from build123d import *

# Parameters (mm, degrees)
SKETCH1_W                   = 90
SKETCH1_H                   = 290
BASE_FLANGE1_DEPTH          = 3
SM_EDGE_FLANGE_1_DEPTH      = 290
SM_EDGE_FLANGE_1_BEND_DEPTH = 290
INDENT1_START               = 23
INDENT1_DEPTH               = 104
INDENT1_START_2             = 26.270388893
INDENT1_2_DEPTH             = 97.459222009
INDENT1_3_DEPTH             = 0.729611107
INDENT1_START_3             = 123
INDENT1_4_DEPTH             = 0.729610902
INDENT1_START_4             = 119.9999999
INDENT1_5_DEPTH             = 6.0000001
INDENT1_START_5             = 24
INDENT1_6_DEPTH             = 6
INDENT1_START_6             = -290
INDENT1_7_DEPTH             = 6.65
INDENT2_START               = 23
INDENT2_DEPTH               = 104
INDENT2_START_2             = -11.0000001
INDENT2_2_DEPTH             = 11.0000001
INDENT2_START_3             = 24
INDENT2_3_DEPTH             = 102
CUT_EXTRUDE1_DEPTH          = 317.754179273
CUT_EXTRUDE1_DEPTH_BACK     = 317.754179273
SKETCH15_R                  = 4.2
CUT_EXTRUDE2_DEPTH          = 317.754179273
CUT_EXTRUDE2_DEPTH_BACK     = 317.754179273


with BuildPart() as part:
    # Base-Flange1: sheet metal written as solids
    # Sketch1 → Base-Flange1 (new body)
    with BuildSketch(Plane(origin=(0, 207.95, 0), x_dir=(1, 0, 0), z_dir=(0, 1, 0))):
        with Locations((75, 145)):
            Rectangle(SKETCH1_W, SKETCH1_H)
    extrude(amount=-BASE_FLANGE1_DEPTH)

    # 邊線-凸緣1: sheet metal written as solids
    # 邊線-凸緣1 section (on a plane across the edge) → 邊線-凸緣1 (add)
    with BuildSketch(Plane(origin=(27, 204.95, 0), x_dir=(1, 0, 0), z_dir=(0, 0, -1))):
        with BuildLine():
            Line((-3, 3), (-3, 15.9))
            Line((-3, 15.9), (0, 15.9))
            Line((0, 15.9), (0, 3))
            ThreePointArc((0, 3), (0.878679656, 0.878679656), (3, 0))
            Line((3, 0), (3, -3))
            ThreePointArc((3, -3), (-1.242640687, -1.242640687), (-3, 3))
        make_face()
    extrude(amount=SM_EDGE_FLANGE_1_DEPTH)

    # 邊線-凸緣1 section 2 (on a plane across the edge) → 邊線-凸緣1 bend (add)
    with BuildSketch(Plane(origin=(123, 204.95, -290), x_dir=(-1, 0, 0), z_dir=(0, 0, 1))):
        with BuildLine():
            Line((-3, 3), (-3, 15.9))
            Line((-3, 15.9), (0, 15.9))
            Line((0, 15.9), (0, 3))
            ThreePointArc((0, 3), (0.878679656, 0.878679656), (3, 0))
            Line((3, 0), (3, -3))
            ThreePointArc((3, -3), (-1.242640687, -1.242640687), (-3, 3))
        make_face()
    extrude(amount=SM_EDGE_FLANGE_1_BEND_DEPTH)

    # Indent1: read off the stored shape, not the designer's step
    # Indent1 outline → Indent1 (cut)
    with BuildSketch(Plane.YZ.offset(INDENT1_START)):
        with BuildLine():
            Line((192.05, -290), (207.95, -290))
            ThreePointArc((207.95, -290), (200, -282.05), (192.05, -290))
        make_face()
    extrude(amount=INDENT1_DEPTH, mode=Mode.SUBTRACT)

    # Indent2: read off the stored shape, not the designer's step
    # Indent2 outline → Indent2 (cut)
    with BuildSketch(Plane.YZ.offset(INDENT2_START)):
        with BuildLine():
            ThreePointArc((189.05, -6.433311744), (197.7062633, -12.491147744), (207.950014124, -9.903902031))
            Line((207.950014124, -9.903902031), (209, -9.061062257))
            Line((209, -9.061062257), (209, 1))
            Line((209, 1), (188, 1))
            Line((188, 1), (188, 0))
            Line((188, 0), (188, -4.64612958))
            Line((188, -4.64612958), (189.05, -6.433311744))
        make_face()
    extrude(amount=INDENT2_DEPTH, mode=Mode.SUBTRACT)

    # Sketch15 → Cut-Extrude1 (cut, two sides: drawn at the far end of the back side and taken through both)
    with BuildSketch(Plane(origin=(0, 207.95, 0), x_dir=(1, 0, 0), z_dir=(0, 1, 0)).offset(-CUT_EXTRUDE1_DEPTH_BACK)):
        with Locations((41.5, 270.8)):
            Circle(SKETCH15_R)
        with Locations((108.5, 270.8)):
            Circle(SKETCH15_R)
        with Locations((41.5, 250.8)):
            Circle(SKETCH15_R)
        with Locations((108.5, 250.8)):
            Circle(SKETCH15_R)
        with Locations((41.5, 230.8)):
            Circle(SKETCH15_R)
        with Locations((108.5, 230.8)):
            Circle(SKETCH15_R)
        with Locations((41.5, 210.8)):
            Circle(SKETCH15_R)
        with Locations((108.5, 210.8)):
            Circle(SKETCH15_R)
        with Locations((41.5, 190.8)):
            Circle(SKETCH15_R)
        with Locations((108.5, 190.8)):
            Circle(SKETCH15_R)
        with Locations((41.5, 170.8)):
            Circle(SKETCH15_R)
        with Locations((108.5, 170.8)):
            Circle(SKETCH15_R)
        with Locations((41.5, 150.8)):
            Circle(SKETCH15_R)
        with Locations((108.5, 150.8)):
            Circle(SKETCH15_R)
        with Locations((41.5, 130.8)):
            Circle(SKETCH15_R)
        with Locations((108.5, 130.8)):
            Circle(SKETCH15_R)
        with Locations((41.5, 110.8)):
            Circle(SKETCH15_R)
        with Locations((108.5, 110.8)):
            Circle(SKETCH15_R)
        with Locations((41.5, 90.8)):
            Circle(SKETCH15_R)
        with Locations((108.5, 90.8)):
            Circle(SKETCH15_R)
        with Locations((41.5, 70.8)):
            Circle(SKETCH15_R)
        with Locations((108.5, 70.8)):
            Circle(SKETCH15_R)
    extrude(amount=CUT_EXTRUDE1_DEPTH + CUT_EXTRUDE1_DEPTH_BACK, mode=Mode.SUBTRACT)

    # Sketch16 → Cut-Extrude2 (cut, two sides: drawn at the far end of the back side and taken through both)
    with BuildSketch(Plane(origin=(0, 207.95, 0), x_dir=(1, 0, 0), z_dir=(0, 1, 0)).offset(-CUT_EXTRUDE2_DEPTH_BACK)):
        with BuildLine():
            Line((55, 54.903913368), (55, 124.903913368))
            ThreePointArc((55, 124.903913368), (75, 144.903913368), (95, 124.903913368))
            Line((95, 124.903913368), (95, 54.903913368))
            ThreePointArc((95, 54.903913368), (75, 34.903913368), (55, 54.903913368))
        make_face()
    extrude(amount=CUT_EXTRUDE2_DEPTH + CUT_EXTRUDE2_DEPTH_BACK, mode=Mode.SUBTRACT)


with BuildPart() as body_2:
    # Indent1 2 outline → Indent1 2 (new body)
    with BuildSketch(Plane.YZ.offset(INDENT1_START_2)):
        with BuildLine():
            Line((204.95, -285.559279338), (204.95, -290))
            Line((204.95, -290), (206.65, -290))
            ThreePointArc((206.65, -290), (206.210475022, -287.622501314), (204.95, -285.559279338))
        make_face()
    extrude(amount=INDENT1_2_DEPTH)

    # Indent1 3 outline → Indent1 3 (add)
    with BuildSketch(Plane.YZ.offset(INDENT1_START_2)):
        with BuildLine():
            Line((193.35, -290), (204.95, -290))
            Line((204.95, -290), (204.95, -285.559279338))
            ThreePointArc((204.95, -285.559279338), (197.622501314, -283.789524978), (193.35, -290))
        make_face()
    extrude(amount=INDENT1_3_DEPTH)

    # Indent1 4 outline → Indent1 4 (add)
    with BuildSketch(Plane.YZ.offset(INDENT1_START_3)):
        with BuildLine():
            Line((193.35, -290), (204.95, -290))
            Line((204.95, -290), (204.95, -285.559279338))
            ThreePointArc((204.95, -285.559279338), (197.622501314, -283.789524978), (193.35, -290))
        make_face()
    extrude(amount=INDENT1_4_DEPTH)

    # Indent1 5 outline → Indent1 5 (add)
    with BuildSketch(Plane.YZ.offset(INDENT1_START_4)):
        with BuildLine():
            Line((193.35, -290), (206.65, -290))
            ThreePointArc((206.65, -290), (200, -283.35), (193.35, -290))
        make_face()
    extrude(amount=INDENT1_5_DEPTH)

    # Indent1 6 outline → Indent1 6 (add)
    with BuildSketch(Plane.YZ.offset(INDENT1_START_5)):
        with BuildLine():
            Line((193.35, -290), (206.65, -290))
            ThreePointArc((206.65, -290), (200, -283.35), (193.35, -290))
        make_face()
    extrude(amount=INDENT1_6_DEPTH)

    # Indent1 7 outline → Indent1 7 (cut)
    with BuildSketch(Plane.XY.offset(INDENT1_START_6)):
        with BuildLine():
            Line((123, 192), (123, 201.95))
            ThreePointArc((123, 201.95), (122.121320344, 204.071320344), (120, 204.95))
            Line((120, 204.95), (119.9999999, 192))
            Line((119.9999999, 192), (123, 192))
        make_face()
        with BuildLine():
            Line((27, 192), (30, 192))
            Line((30, 192), (30, 204.95))
            ThreePointArc((30, 204.95), (27.878679656, 204.071320344), (27, 201.95))
            Line((27, 201.95), (27, 192))
        make_face()
        with BuildLine():
            ThreePointArc((123.729603466, 206.650006169), (125.402666971, 204.559825589), (126, 201.95))
            Line((126, 201.95), (126, 208))
            Line((126, 208), (122.028355761, 208))
            Line((122.028355761, 208), (123.729603466, 206.650006169))
        make_face()
        with BuildLine():
            Line((24, 208), (24, 201.95))
            ThreePointArc((24, 201.95), (24.597331636, 204.559822705), (26.270391517, 206.650002187))
            Line((26.270391517, 206.650002187), (27.971640511, 208))
            Line((27.971640511, 208), (24, 208))
        make_face()
    extrude(amount=INDENT1_7_DEPTH, mode=Mode.SUBTRACT)


with BuildPart() as body_3:
    # Indent2 2 outline → Indent2 2 (new body)
    with BuildSketch(Plane.XY.offset(INDENT2_START_2)):
        with BuildLine():
            Line((24, 201.95), (24, 189.05))
            Line((24, 189.05), (27, 189.05))
            Line((27, 189.05), (27, 201.95))
            ThreePointArc((27, 201.95), (27.878679656, 204.071320344), (30, 204.95))
            Line((30, 204.95), (120, 204.95))
            ThreePointArc((120, 204.95), (122.121320344, 204.071320344), (123, 201.95))
            Line((123, 201.95), (123, 189.05))
            Line((123, 189.05), (126, 189.05))
            Line((126, 189.05), (126, 201.95))
            ThreePointArc((126, 201.95), (124.242640687, 206.192640687), (120, 207.95))
            Line((120, 207.95), (30, 207.95))
            ThreePointArc((30, 207.95), (25.757359313, 206.192640687), (24, 201.95))
        make_face()
    extrude(amount=INDENT2_2_DEPTH)

    # Indent2 3 outline → Indent2 3 (cut)
    with BuildSketch(Plane.YZ.offset(INDENT2_START_3)):
        with BuildLine():
            Line((207.95, -11.0000001), (207.950016725, -7.602449216))
            ThreePointArc((207.950016725, -7.602449216), (204.322791843, -10.115012145), (200.000000001, -11))
            Line((200.000000001, -11), (207.95, -11.0000001))
        make_face()
        with BuildLine():
            Line((189.05, -11.0000001), (200.000000001, -11))
            ThreePointArc((200.000000001, -11), (192.601479194, -8.140140655), (189.05, -1.047616342))
            Line((189.05, -1.047616342), (189.05, -11.0000001))
        make_face()
    extrude(amount=INDENT2_3_DEPTH, mode=Mode.SUBTRACT)


solid = part.part
Here's how the part is built. I have some questions about the finished solid (model axes, mm). A direction names the side the tool comes from. Coordinates: 2 decimals unless noted, no trailing zeros. Write each loop counter-clockwise with the first axis right and the second up, starting at its lowest first coordinate (ties: lowest second). Pieces come first, ordered by that corner, then holes.
1) I'm going to push flat-ended pins straight in: pin 1 (11 mm diameter, centred on x = 41.5, z = -150.8, fed in from +Y); pin 2 (0.9 mm diameter, centred on y = 206.5, z = -82, fed in from +X); pin 3 (1 mm diameter, centred on x = 76.5, z = -243, fed in from -Y); pin 4 (1.5 mm diameter, centred on y = 207, z = -105, fed in from -X). Where does each tip first touch, or does it pass through?
Filled in:
pin 1: stops at y = 207.95
pin 2: stops at x = 124.38
pin 3: stops at y = 204.95
pin 4: stops at x = 25.82
2) If we section it at D-D (x = 67): List the corners of the cut face in (y, z) for me, plus the area to 3 significant figures.
Filled in:
outline: (204.95, -283.78) arc R7.95 cw to (207.95, -290) - (207.95, -143.23) - (204.95, -143.23) - close; (204.95, -36.57) - (207.95, -36.57) - (207.95, -9.9) arc R12.7 cw to (204.95, -11.7) - close
area: 504 mm2
3) If we section it at B-B (y = 196): List the corners of the cut face in (x, z) for me, plus the area to 3 significant figures.
Filled in:
outline: (24, -283.13) - (27, -283.13) - (27, -12.05) - (24, -12.05) - close; (123, -283.13) - (126, -283.13) - (126, -12.05) - (123, -12.05) - close
area: 1,630 mm2
4) If we section it at C-C (z = -44.5): List the corners of the cut face in (x, y) for me.
Filled in:
outline: (24, 189.05) - (27, 189.05) - (27, 201.95) arc R3 cw to (30, 204.95) - (57.92, 204.95) - (57.92, 207.95) - (30, 207.95) arc R6 ccw to (24, 201.95) - close; (92.08, 204.95) - (120, 204.95) arc R3 cw to (123, 201.95) - (123, 189.05) - (126, 189.05) - (126, 201.95) arc R6 ccw to (120, 207.95) - (92.08, 207.95) - close
5) If we section it at A-A (z = -170.8): List the corners of the cut face in (x, y) for me, plus the area to 3 significant figures.
Filled in:
outline: (24, 189.05) - (27, 189.05) - (27, 201.95) arc R3 cw to (30, 204.95) - (37.3, 204.95) - (37.3, 207.95) - (30, 207.95) arc R6 ccw to (24, 201.95) - close; (45.7, 204.95) - (104.3, 204.95) - (104.3, 207.95) - (45.7, 207.95) - close; (112.7, 204.95) - (120, 204.95) arc R3 cw to (123, 201.95) - (123, 189.05) - (126, 189.05) - (126, 201.95) arc R6 ccw to (120, 207.95) - (112.7, 207.95) - close
area: 339 mm2
6) Which directions (+Z, -Z, +X, -X, +Y, -Y) give clear straight access to the entire face, cutting with the end or side of a thin tool? Please do faces 4 (the face through (123, 195, -150)), 5 (the face through (75.44, 206.43, -34.91)).
Filled in:
face 4: +Z, -Z, -Y
face 5: +Y, -Y
7) Thinking about a two-plate mould opening in Z: for faces 1 (the face through (126, 196, -150)), 2 (the face through (112.38, 206.43, -109.19)), 3 (the face through (74.762, 206.914, -286.076)), which applies, +Z half, -Z half, draft (parallel to the pull), parting line (faces both ways), or undercut?
Filled in:
face 1: draft
face 2: undercut
face 3: -Z half
8) If I drill on line 1 (X direction, y = 191, z = -273); line 2 (X direction, y = 202.5, z = -46.5); line 3 (Y direction, x = 45.5, z = -143), over which ranges is the centre line in solid material (lowest first)?
Filled in:
line 1: x = 24 to 27, 123 to 126
line 2: x = 24.03 to 27.05, 122.95 to 125.97
line 3: y = 204.95 to 207.95
